```python
from build123d import *

# Parameters (mm, degrees)
SZKIC1_W                    = 4.44
SZKIC1_H                    = 33.58
DODANIE_WYCI_GNI_CIE1_DEPTH = 1
SZKIC2_W                    = 0.64
SZKIC2_H                    = 0.64
WYTNIJ_WYCI_GNI_CIE1_DEPTH  = 1
SZKIC3_W                    = 1
SZKIC3_H                    = 0.25
DODANIE_WYCI_GNI_CIE2_DEPTH = 1
SZKIC4_W                    = 4.44
SZKIC4_H                    = 1
DODANIE_WYCI_GNI_CIE3_DEPTH = 4
SZKIC5_W                    = 1
SZKIC5_H                    = 0.25
DODANIE_WYCI_GNI_CIE4_DEPTH = 1
SZKIC6_W                    = 1
SZKIC6_H                    = 1
WYTNIJ_WYCI_GNI_CIE2_DEPTH  = 4


with BuildPart() as part:
    # Szkic1 → Dodanie-wyciągnięcie1 (new body)
    with BuildSketch(Plane(origin=(0, 0, 0), x_dir=(1, 0, 0), z_dir=(0, 1, 0))):
        Rectangle(SZKIC1_W, SZKIC1_H)
    extrude(amount=DODANIE_WYCI_GNI_CIE1_DEPTH)

    # Szkic2 → Wytnij-wyciągnięcie1 (cut)
    with BuildSketch(Plane(origin=(0, 1, 0), x_dir=(1, 0, 0), z_dir=(0, 1, 0))):
        with Locations((0, -13.97)):
            Rectangle(SZKIC2_W, SZKIC2_H)
        with Locations((0, -11.43)):
            Rectangle(SZKIC2_W, SZKIC2_H)
        with Locations((0, -8.89)):
            Rectangle(SZKIC2_W, SZKIC2_H)
        with Locations((0, -6.35)):
            Rectangle(SZKIC2_W, SZKIC2_H)
        with Locations((0, -3.81)):
            Rectangle(SZKIC2_W, SZKIC2_H)
        with Locations((0, -1.27)):
            Rectangle(SZKIC2_W, SZKIC2_H)
        with Locations((0, 1.27)):
            Rectangle(SZKIC2_W, SZKIC2_H)
        with Locations((0, 3.81)):
            Rectangle(SZKIC2_W, SZKIC2_H)
        with Locations((0, 6.35)):
            Rectangle(SZKIC2_W, SZKIC2_H)
        with Locations((0, 8.89)):
            Rectangle(SZKIC2_W, SZKIC2_H)
        with Locations((0, 11.43)):
            Rectangle(SZKIC2_W, SZKIC2_H)
        with Locations((0, 13.97)):
            Rectangle(SZKIC2_W, SZKIC2_H)
    extrude(amount=-WYTNIJ_WYCI_GNI_CIE1_DEPTH, mode=Mode.SUBTRACT)

    # Szkic3 → Dodanie-wyciągnięcie2 (add)
    with BuildSketch(Plane.XZ):
        with Locations((0, 16.0350189)):
            Rectangle(SZKIC3_W, SZKIC3_H)
    extrude(amount=DODANIE_WYCI_GNI_CIE2_DEPTH)

    # Szkic4 → Dodanie-wyciągnięcie3 (add)
    with BuildSketch(Plane.XZ):
        with Locations((0, -16.29)):
            Rectangle(SZKIC4_W, SZKIC4_H)
    extrude(amount=DODANIE_WYCI_GNI_CIE3_DEPTH)

    # Szkic5 → Dodanie-wyciągnięcie4 (add)
    with BuildSketch(Plane.XZ.offset(4)):
        with Locations((0, -16.29)):
            Rectangle(SZKIC5_W, SZKIC5_H)
    extrude(amount=DODANIE_WYCI_GNI_CIE4_DEPTH)

    # Szkic6 → Wytnij-wyciągnięcie2 (cut)
    with BuildSketch(Plane.XZ.offset(4)):
        with Locations((1.72, -16.29)):
            Rectangle(SZKIC6_W, SZKIC6_H)
        with Locations((-1.72, -16.29)):
            Rectangle(SZKIC6_W, SZKIC6_H)
    extrude(amount=-WYTNIJ_WYCI_GNI_CIE2_DEPTH, mode=Mode.SUBTRACT)


solid = part.part
```
The model under review builds one solid part; all positions refer to its coordinate system, in mm. A direction names the side the tool comes from. Round coordinates to 2 decimals unless told otherwise and drop trailing zeros. Write each loop counter-clockwise with the first axis right and the second up, starting at its lowest first coordinate (ties: lowest second). Pieces come first, ordered by that corner, then holes. Notation, with made-up numbers: (38, 9) - (53, 9) arc R26 cw to (53, 31) - close; hole circle Ø2 at (49.25, 72.25). An arc over 180 degrees is marked (long way). Answer as CSV lines item,"result". Start each with the question number.
(1) We need section B-B on x = -1.65. State the section outline as (y, z) points, plus the area to 3 significant figures.
(2) To check wall thickness, follow line 1 (Y direction, x = -1.9, z = -11); line 2 (Z direction, x = 0.15, y = -0.3); line 3 (Z direction, x = 0.5, y = -2.2). State the ranges of each line that lie inside material, in increasing order.
(3) For faces 5 (the flat face through (0, -0.5, 16.16)), 6 (the flat face through (0, -4.5, -16.415)), 7 (the flat face through (1.22, -2, -16)), 8 (the flat face through (-1.22, -2, -16)), list the 3-axis set-ups (+Z, -Z, +X, -X, +Y, -Y) from which the entire face can be reached by the end or side of a thin tool; tool diameter is ignored.
(4) We need section A-A on y = -0.5. State the section outline as (x, z) points, plus the area to 3 significant figures.
(5) Draft analysis for pull direction Z (two halves, no side actions). For faces 1 (the flat face through (0, -0.5, 15.91)), 2 (the flat face through (0, 0, 0)), 3 (the flat face through (0, -4, -16)), 4 (the flat face through (0, 0.5, 16.79)), state which applies: pulls with the +Z half, pulls with the -Z half, needs draft (parallel to the pull), parting line crosses it, or undercut.
(6) We need section C-C on z = -8. State the section outline as (x, y) points.
(7) For pin 1 Ø2 at (x, z) = (0.5, 0.5) entering from -Y; pin 2 Ø2 at (y, z) = (-0.5, 7.5) entering from -X; pin 3 Ø0.8 at (y, z) = (-1.5, -16.5) entering from +X; pin 4 Ø1.2 at (x, y) = (0, -2.5) entering from +Z, all flat-tipped, find the tip position at first contact; note any pin that passes through.
Worked answers:
1,outline,"(0, -16.79) - (1, -16.79) - (1, 16.79) - (0, 16.79) - close"
1,area,"33.6 mm²"
2,line 1,"0 to 1"
2,line 2,"-16.79 to -15.79, 15.91 to 16.16"
2,line 3,"-16.79 to -15.79"
3,face 5,"+Z, +X, -X, -Y"
3,face 6,"-Z, +X, -X, -Y"
3,face 7,"+Z, -Z, +X, -Y"
3,face 8,"+Z, -Z, -X, -Y"
4,outline,"(-1.22, -16.79) - (1.22, -16.79) - (1.22, -15.79) - (-1.22, -15.79) - close; (-0.5, 15.91) - (0.5, 15.91) - (0.5, 16.16) - (-0.5, 16.16) - close"
4,area,"2.69 mm²"
5,face 1,"undercut"
5,face 2,"undercut"
5,face 3,"needs draft"
5,face 4,"pulls with the +Z half"
6,outline,"(-2.22, 0) - (2.22, 0) - (2.22, 1) - (-2.22, 1) - close"
7,pin 1,"y = 0"
7,pin 2,"x = -2.22"
7,pin 3,"x = 1.22"
7,pin 4,"z = -15.79"
